Geometry: final body of the model. Coordinates: model frame, mm. Face numbers are marked on the shaded views. A direction names the side the tool comes from. Round coordinates to 2 decimals unless told otherwise and drop trailing zeros. Loops run counter-clockwise (first coordinate to the right, second up) from the corner with the lowest first, then second, coordinate; pieces in that order, holes last. Notation, with made-up numbers: M 58,25.25 L 68,25.25 A24 ccw 68,38.25 Z; hole C 58.5,85 d8. An arc over 180 degrees is marked long. Answer as a JSON object with one key per item and string values.
from build123d import *

# Parameters (mm, degrees)
F0_R     = 18.25625
F1_DEPTH = 6.35
F2_R     = 16.66875
F3_DEPTH = 68.2625
F4_R     = 1.58749


# Not quite as in the source:
# - a fillet or chamfer is up to 0.001 mm smaller than in the source, because OpenCascade refuses the exact size


with BuildPart() as f1:
    # F0 (on Top) → F1 (new body)
    with BuildSketch(Plane.XY):
        Circle(F0_R)
    extrude(amount=F1_DEPTH)

    # F2 (on face) → F3 (join)
    with BuildSketch(Plane.XY.offset(6.35)):
        Circle(F2_R)
    extrude(amount=F3_DEPTH)

    # F4 (radius 1.5875 in the source; OpenCascade refuses exactly that, so slightly less here)
    f4_edges = [f1.edges().sort_by_distance(p)[0] for p in [
        (-18.25625, 0, 6.35),
        (-16.66875, 0, 74.6125),
    ]]
    fillet(f4_edges, radius=F4_R)


solid = f1.part
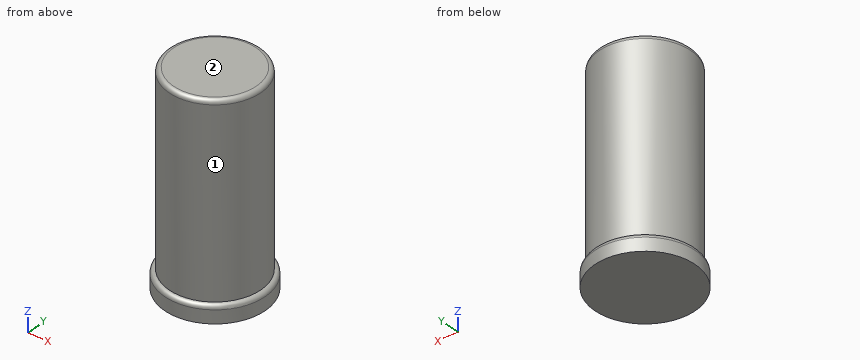
1) Pin query (flat end, axial travel): P1, Ø6, axis at y = 3.5, z = 39, coming from the -X side; P2, Ø2, axis at x = -9.5, z = 22, coming from the +Y side; P3, Ø5, axis at x = 5.5, z = 42, coming from the +Y side. Return the tip coordinate at first contact, or that it passes through.
Results:
{"P1": "x = -16.66", "P2": "y = 14.34", "P3": "y = 16.4"}
2) Ray query, line 1 (Z direction, x = 10, y = -13.5); line 2 (Y direction, x = -11, z = 16); line 3 (Z direction, x = 14.5, y = 9.5). Return the intervals inside material, ascending.
Results:
{"line 1": "0 to 6.34", "line 2": "-12.52 to 12.52", "line 3": "0 to 6.2"}
3) Reachability of the marked faces 1 and 2 from +Z, -Z, +X, -X, +Y, -Y: full face, straight path, thin tool, end or side. Return the list, or none.
Results:
{"face 1": "+Z", "face 2": "+Z, +X, -X, +Y, -Y"}
4) Section query C-C (z = 16). Return the cut outline in (x, y), and give its area (3 significant figures).
Results:
{"outline": "C 0,0 d33.34", "area": "873 mm2"}
